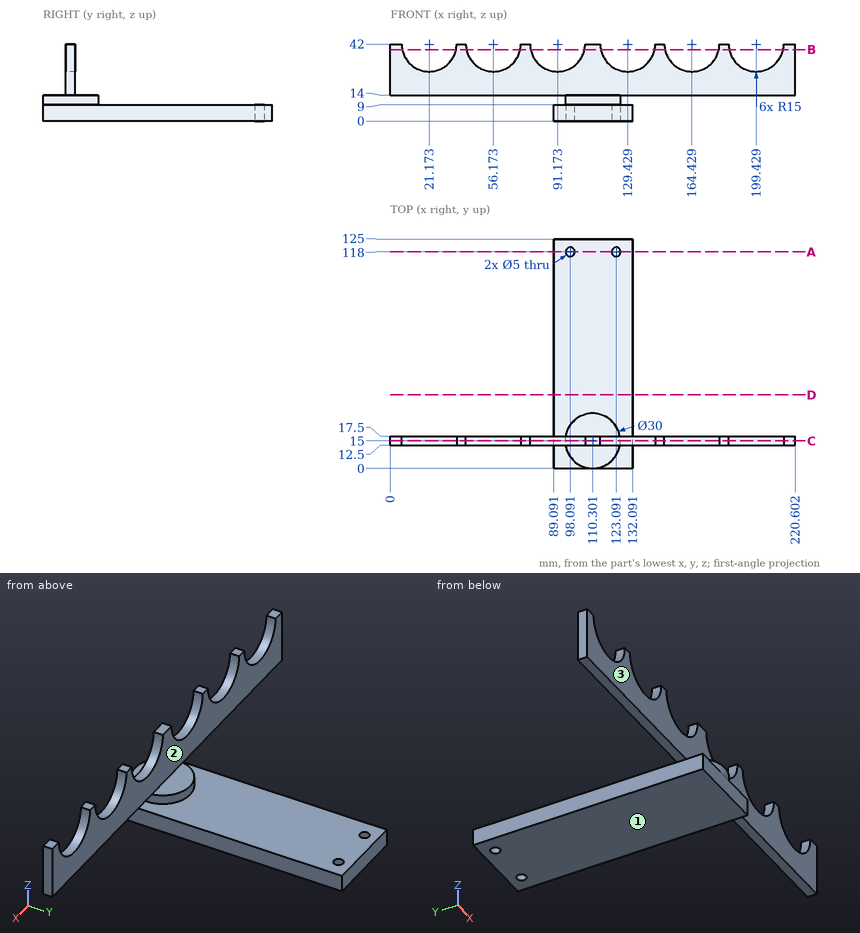
Study the drawing (mm; zero at the part's minimum x, y, z) and answer. A direction names the side the tool comes from. Coordinates: 2 decimals unless noted, no trailing zeros. Order: outer loops, then holes, each group sorted by start corner. A loop starts at its lowest first (then second) coordinate and runs counter-clockwise, first axis right, second up. Notation, with made-up numbers: (19, 88.25) -> (52, 88.25) arc R29 ccw to (52, 126.25) -> close; hole circle Ø5 at (-1.5, 69). An arc over 180 degrees is marked (long way). Answer in a Markdown table with one row per item. Add a question column.
Item 1: Find section C-C (y = 15). Write down the section's boundary in (x, z), then the cut area to 3 significant figures.
Item 2: Find section D-D (y = 40). Write down the section's boundary in (x, z), then the cut area to 3 significant figures.
Item 3: Find section B-B (z = 39). Write down the section's boundary in (x, y) (1 decimal), then the cut area to 3 significant figures.
Item 4: Find section A-A (y = 118). Write down the section's boundary in (x, z), then the cut area to 3 significant figures.
Item 5: Find the intervals of material crossed by L1, parallel to X at y = 7.5, z = 2.5; L2, parallel to Z at x = 105.5, y = 53; L3, parallel to Y at x = 182.5, z = 39, in increasing order. Write a range as from..to.
Item 6: Each of these flat-tipped pins is pushed along its axis until it touches: P1, Ø1, axis at x = 107, z = 21.5, coming from the +Y side; P2, Ø4, axis at x = 106, y = 5.5, coming from the +Z side; P3, Ø14, axis at x = 163, z = 31, coming from the -Y side. Where does it stop, or does it pass through?
Item 7: Which of the six approach directions +Z, -Z, +X, -X, +Y, -Y give full straight-line access (tool end or side, diameter ignored) to the marked faces 1, 2 and 3?
Result set:
| question | item | result |
|---|---|---|
| 1 | outline | (0, 14) -> (95.3, 14) -> (95.3, 9) -> (89.09, 9) -> (89.09, 0) -> (132.09, 0) -> (132.09, 9) -> (125.3, 9) -> (125.3, 14) -> (220.6, 14) -> (220.6, 42) -> (214.43, 42) arc R15 cw to (184.43, 42) -> (179.43, 42) arc R15 cw to (149.43, 42) -> (144.43, 42) arc R15 cw to (114.43, 42) -> (106.17, 42) arc R15 cw to (76.17, 42) -> (71.17, 42) arc R15 cw to (41.17, 42) -> (36.17, 42) arc R15 cw to (6.17, 42) -> (0, 42) -> close |
| 1 | area | 4,590 mm² |
| 2 | outline | (89.09, 0) -> (132.09, 0) -> (132.09, 9) -> (89.09, 9) -> close |
| 2 | area | 387 mm² |
| 3 | outline | (0, 12.5) -> (6.5, 12.5) -> (6.5, 17.5) -> (0, 17.5) -> close; (35.9, 12.5) -> (41.5, 12.5) -> (41.5, 17.5) -> (35.9, 17.5) -> close; (70.9, 12.5) -> (76.5, 12.5) -> (76.5, 17.5) -> (70.9, 17.5) -> close; (105.9, 12.5) -> (114.7, 12.5) -> (114.7, 17.5) -> (105.9, 17.5) -> close; (144.1, 12.5) -> (149.7, 12.5) -> (149.7, 17.5) -> (144.1, 17.5) -> close; (179.1, 12.5) -> (184.7, 12.5) -> (184.7, 17.5) -> (179.1, 17.5) -> close; (214.1, 12.5) -> (220.6, 12.5) -> (220.6, 17.5) -> (214.1, 17.5) -> close |
| 3 | area | 221 mm² |
| 4 | outline | (89.09, 0) -> (95.59, 0) -> (95.59, 9) -> (89.09, 9) -> close; (100.59, 0) -> (120.59, 0) -> (120.59, 9) -> (100.59, 9) -> close; (125.59, 0) -> (132.09, 0) -> (132.09, 9) -> (125.59, 9) -> close |
| 4 | area | 297 mm² |
| 5 | L1 | x = 89.09..132.09 |
| 5 | L2 | z = 0..9 |
| 5 | L3 | y = 12.5..17.5 |
| 6 | P1 | stops at y = 17.5 |
| 6 | P2 | stops at z = 14 |
| 6 | P3 | stops at y = 12.5 |
| 7 | face 1 | -Z, +X, -X, +Y, -Y |
| 7 | face 2 | +Z, +X, -X, +Y |
| 7 | face 3 | +Z, +X, -X, -Y |
